```python
from build123d import *

# Parameters (mm, degrees)
F0_W     = 30.48
F0_H     = 32.512
F0_R     = 8.50011
F0_W_2   = 1.4986
F0_H_2   = 14.5034
F1_DEPTH = 2.794
F2_SIZE  = 1.4224
F3_SIZE  = 1.4224
F4_SIZE  = 1.4224
F5_SIZE  = 1.4224
F6_R     = 0.635
F7_R     = 0.635
F8_R     = 0.635
F9_R     = 0.635


with BuildPart() as f1:
    # F0 (on Right) → F1 (new body)
    with BuildSketch(Plane.YZ):
        with Locations((42.135775, 10.835214)):
            Rectangle(F0_W, F0_H)
        with Locations((39.595775, 10.939535)):
            Circle(F0_R, mode=Mode.SUBTRACT)
        with Locations((54.315075, 10.835214)):
            Rectangle(F0_W_2, F0_H_2, mode=Mode.SUBTRACT)
    extrude(amount=F1_DEPTH)

    # F2
    f2_edges = [f1.edges().sort_by_distance(p)[0] for p in [
        (1.397, 57.375775, 27.091214),
    ]]
    chamfer(f2_edges, length=F2_SIZE)

    # F3
    f3_edges = [f1.edges().sort_by_distance(p)[0] for p in [
        (1.397, 26.895775, 27.091214),
    ]]
    chamfer(f3_edges, length=F3_SIZE)

    # F4
    f4_edges = [f1.edges().sort_by_distance(p)[0] for p in [
        (1.397, 26.895775, -5.420786),
    ]]
    chamfer(f4_edges, length=F4_SIZE)

    # F5
    f5_edges = [f1.edges().sort_by_distance(p)[0] for p in [
        (1.397, 57.375775, -5.420786),
    ]]
    chamfer(f5_edges, length=F5_SIZE)

    # F6
    f6_edges = [f1.edges().sort_by_distance(p)[0] for p in [
        (1.397, 53.565775, 3.583514),
    ]]
    fillet(f6_edges, radius=F6_R)

    # F7
    f7_edges = [f1.edges().sort_by_distance(p)[0] for p in [
        (1.397, 55.064375, 3.583514),
    ]]
    fillet(f7_edges, radius=F7_R)

    # F8
    f8_edges = [f1.edges().sort_by_distance(p)[0] for p in [
        (1.397, 53.565775, 18.086914),
    ]]
    fillet(f8_edges, radius=F8_R)

    # F9
    f9_edges = [f1.edges().sort_by_distance(p)[0] for p in [
        (1.397, 55.064375, 18.086914),
    ]]
    fillet(f9_edges, radius=F9_R)


solid = f1.part
```
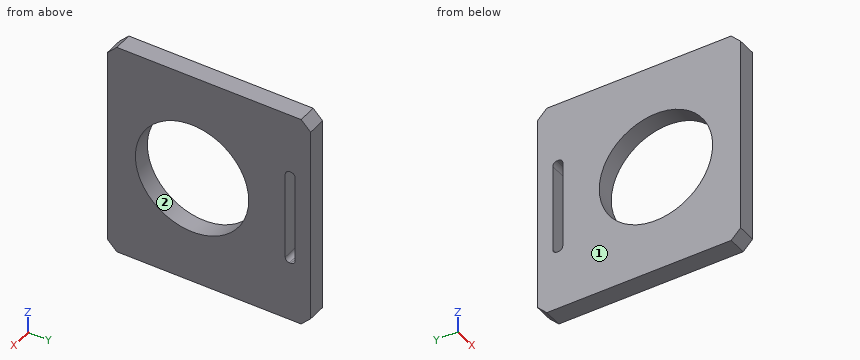
Geometry: final body of the model. Coordinates: model frame, mm. Face numbers are marked on the shaded views. Round coordinates to 2 decimals unless told otherwise and drop trailing zeros. Order: outer loops, then holes, each group sorted by start corner. A loop starts at its lowest first (then second) coordinate and runs counter-clockwise, first axis right, second up. Notation, with made-up numbers: (65, 37.25) - (87, 37.25) arc R17 cw to (87, 70.25) - close; hole circle Ø6 at (89.5, 23.5). An arc over 180 degrees is marked (long way). Use CSV: the item, a comma, the result in double quotes. Start each with the question number.
Q1. Section query B-B (x = 1.75). Return loops of the section in (y, z) (3 decimals), and give its area (3 significant figures).
Q2. Material intervals for line 1 along Y through (x, z) = (2.6, 10); line 2 along Y through (x, z) = (1.6, 6); line 3 along Z through (x, y) = (2.6, 54.5), sorted ascending. Write a range as from..to.
Q3. Mould query, pull axis Y, two halves, no side actions, for the marked faces 1 and 2. Classes: +Y half, -Y half, draft (parallel to the pull), parting line (faces both ways), or undercut.
Q4. Section query D-D (z = 15.5). Return loops of the section in (x, y).
Q5. Section query C-C (z = 11.5). Return loops of the section in (x, y).
Q6. Section query A-A (y = 41.5). Return loops of the section in (x, z).
Result set:
1,outline,"(26.896, -3.998) - (28.318, -5.421) - (55.953, -5.421) - (57.376, -3.998) - (57.376, 25.669) - (55.953, 27.091) - (28.318, 27.091) - (26.896, 25.669) - close; hole circle Ø17 at (39.596, 10.94); hole (53.566, 4.219) arc R0.635 ccw to (54.201, 3.584) - (54.429, 3.584) arc R0.635 ccw to (55.064, 4.219) - (55.064, 17.452) arc R0.635 ccw to (54.429, 18.087) - (54.201, 18.087) arc R0.635 ccw to (53.566, 17.452) - close"
1,area,"739 mm2"
2,line 1,"y = 26.9..31.15, 48.04..53.57, 55.06..57.38"
2,line 2,"y = 26.9..32.68, 46.51..53.57, 55.06..57.38"
2,line 3,"z = -5.42..3.59, 18.08..27.09"
3,face 1,"draft"
3,face 2,"undercut"
4,outline,"(0, 26.9) - (2.79, 26.9) - (2.79, 32.42) - (0, 32.42) - close; (0, 46.77) - (2.79, 46.77) - (2.79, 53.57) - (0, 53.57) - close; (0, 55.06) - (2.79, 55.06) - (2.79, 57.38) - (0, 57.38) - close"
5,outline,"(0, 26.9) - (2.79, 26.9) - (2.79, 31.11) - (0, 31.11) - close; (0, 48.08) - (2.79, 48.08) - (2.79, 53.57) - (0, 53.57) - close; (0, 55.06) - (2.79, 55.06) - (2.79, 57.38) - (0, 57.38) - close"
6,outline,"(0, -5.42) - (2.79, -5.42) - (2.79, 2.66) - (0, 2.66) - close; (0, 19.22) - (2.79, 19.22) - (2.79, 27.09) - (0, 27.09) - close"
